from build123d import *

# Parameters (mm, degrees)
F1_DEPTH  = 27
F3_DEPTH  = 25
F5_DEPTH  = 5
F6_R      = 3
F7_R      = 3
F9_R      = 0.75
F10_DEPTH = 5


with BuildPart() as f1:
    # F0 (on Top) → F1 (new body)
    with BuildSketch(Plane.XY):
        with BuildLine():
            Line((76, 0), (10, 0))
            ThreePointArc((10, 0), (2.928932, -2.928932), (0, -10))
            Line((0, -10), (0, -56))
            ThreePointArc((0, -56), (2.928932, -63.071068), (10, -66))
            Line((10, -66), (76, -66))
            ThreePointArc((76, -66), (83.071068, -63.071068), (86, -56))
            Line((86, -56), (86, -10))
            ThreePointArc((86, -10), (83.071068, -2.928932), (76, 0))
        make_face()
    extrude(amount=F1_DEPTH)

    # F2 (on face) → F3 (cut)
    with BuildSketch(Plane.XY.offset(27)):
        with BuildLine():
            Line((73, -3), (13, -3))
            ThreePointArc((13, -3), (5.928932, -5.928932), (3, -13))
            Line((3, -13), (3, -53))
            ThreePointArc((3, -53), (5.928932, -60.071068), (13, -63))
            Line((13, -63), (73, -63))
            ThreePointArc((73, -63), (80.071068, -60.071068), (83, -53))
            Line((83, -53), (83, -13))
            ThreePointArc((83, -13), (80.071068, -5.928932), (73, -3))
        make_face()
    extrude(amount=-F3_DEPTH, mode=Mode.SUBTRACT)

    # F4 (on face) → F5 (cut)
    with BuildSketch(Plane.XY.offset(27)):
        with BuildLine():
            Line((74.7, -1.3), (11.3, -1.3))
            ThreePointArc((11.3, -1.3), (4.228932, -4.228932), (1.3, -11.3))
            Line((1.3, -11.3), (1.3, -54.7))
            ThreePointArc((1.3, -54.7), (4.228932, -61.771068), (11.3, -64.7))
            Line((11.3, -64.7), (74.7, -64.7))
            ThreePointArc((74.7, -64.7), (81.771068, -61.771068), (84.7, -54.7))
            Line((84.7, -54.7), (84.7, -11.3))
            ThreePointArc((84.7, -11.3), (81.771068, -4.228932), (74.7, -1.3))
        make_face()
    extrude(amount=-F5_DEPTH, mode=Mode.SUBTRACT)

    # F6
    f6_edges = [f1.edges().sort_by_distance(p)[0] for p in [
        (43, 0, 0),
        (2.928932, -2.928932, 0),
        (0, -33, 0),
        (83.071068, -2.928932, 0),
        (86, -33, 0),
        (83.071068, -63.071068, 0),
        (43, -66, 0),
        (2.928932, -63.071068, 0),
    ]]
    fillet(f6_edges, radius=F6_R)

    # F7
    f7_edges = [f1.edges().sort_by_distance(p)[0] for p in [
        (43, -3, 2),
    ]]
    fillet(f7_edges, radius=F7_R)

    # F9 (on offset) → F10 (join, symmetric)
    with BuildSketch(Plane.YZ.offset(43)):
        with Locations((-1.3, 24.5)):
            Circle(F9_R)
        with Locations((-64.7, 24.5)):
            Circle(F9_R)
    extrude(amount=F10_DEPTH, both=True)


solid = f1.part
Design review of the part built by this model. Coordinates are the model's own, in mm. A direction names the side the tool comes from. Coordinates: 2 decimals unless noted, no trailing zeros. Order: outer loops, then holes, each group sorted by start corner. A loop starts at its lowest first (then second) coordinate and runs counter-clockwise, first axis right, second up.
Item 1: For faces 4 (the cylindrical face through (80.15, -6.01, 13.62)), 5 (the cylindrical face through (0.86, -33.32, 0.9)), list the 3-axis set-ups (+Z, -Z, +X, -X, +Y, -Y) from which the entire face can be reached by the end or side of a thin tool; tool diameter is ignored.
Item 2: For line 1 (X direction, y = -47.5, z = 14.25); line 2 (Y direction, x = 61, z = 16.75); line 3 (X direction, y = -19, z = 22.25), list the stretches that pass through material, from the lowest coordinate up.
Item 3: The part is to be moulded in two halves that separate along X. For faces 1 (the flat face through (33.5, -63.4, 22)), 2 (the cylindrical face through (42.54, -0.86, 0.9)), 3 (the flat face through (86, -33, 15)), say which applies: pulls with the +X half, pulls with the -X half, needs draft (parallel to the pull), parting line crosses it, or undercut.
Item 4: Take a section at C-C, the plane z = 4. Write out the cut boundary in (x, y), then the cut area to 3 significant figures.
Item 5: For pin 1 Ø1 at (x, y) = (19.5, -41) entering from +Z; pin 2 Ø0.6 at (y, z) = (-1.5, 24.5) entering from -X; pin 3 Ø0.6 at (y, z) = (-64, 24) entering from +X, all flat-tipped, find the tip position at first contact; note any pin that passes through.
Item 6: Take a section at B-B, the plane y = -44. Write out the cut boundary in (x, z).
Item 7: Take a section at A-A, the plane x = 62. Write out the cut boundary in (y, z), then the cut area to 3 significant figures.
The answers:
1. face 4: +Z
1. face 5: -Z, -X, +Y, -Y
2. line 1: x = 0 to 3, 83 to 86
2. line 2: y = -66 to -63, -3 to 0
2. line 3: x = 0 to 1.3, 84.7 to 86
3. face 1: undercut
3. face 2: needs draft
3. face 3: pulls with the +X half
4. outline: (0, -56) arc R10 ccw to (10, -66) - (76, -66) arc R10 ccw to (86, -56) - (86, -10) arc R10 ccw to (76, 0) - (10, 0) arc R10 ccw to (0, -10) - close; hole (3.17, -53) arc R9.83 ccw to (13, -62.83) - (73, -62.83) arc R9.83 ccw to (82.83, -53) - (82.83, -13) arc R9.83 ccw to (73, -3.17) - (13, -3.17) arc R9.83 ccw to (3.17, -13) - close
4. area: 921 mm2
5. pin 1: stops at z = 2
5. pin 2: stops at x = 4.28
5. pin 3: stops at x = 82.38
6. outline: (0, 3) arc R3 ccw to (3, 0) - (83, 0) arc R3 ccw to (86, 3) - (86, 27) - (84.7, 27) - (84.7, 22) - (83, 22) - (83, 5) arc R3 cw to (80, 2) - (6, 2) arc R3 cw to (3, 5) - (3, 22) - (1.3, 22) - (1.3, 27) - (0, 27) - close
7. outline: (-66, 3) arc R3 ccw to (-63, 0) - (-3, 0) arc R3 ccw to (0, 3) - (0, 27) - (-1.3, 27) - (-1.3, 22) - (-3, 22) - (-3, 5) arc R3 cw to (-6, 2) - (-60, 2) arc R3 cw to (-63, 5) - (-63, 22) - (-64.7, 22) - (-64.7, 27) - (-66, 27) - close
7. area: 265 mm2
